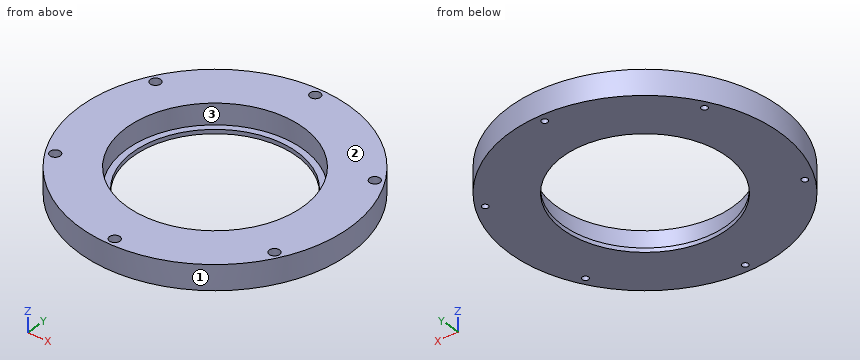
Autodesk Fusion 360 part; units mm, degrees
sketch "Sketch1" plane through (0, 0, 0) normal (0, 0, 1) x (1, 0, 0)
  circle A0 centre (0, 0) radius 65
  circle A1 centre (0, 0) radius 61.0225 construction
  circle A2 centre (0, 0) radius 39.5
  circle A3 centre (0, -61.0225) radius 1.5
  dimension "d1" = 130
  dimension "d2" = 122.045
  dimension "d3" = 79
  dimension "ScrewDia" = 3
extrude "Extrude1" add sketch "Sketch1" along normal blind 2 contours A0 | A3
sketch "Sketch2" plane through (0, 0, 2) normal (0, 0, 1) x (-1, 0, 0)
  circle A0 centre (0, 0) radius 39.5
  circle A1 centre (0, 0) radius 65
  circle A2 centre (0, 0) radius 42.5
  dimension "BearingDia" = 85
extrude "Extrude2" add sketch "Sketch2" along normal blind 10 contours A1
extrude "Extrude3" cut sketch "Sketch1" along normal blind 25 contours A3
sketch "Sketch3" plane through (0, 0, 12) normal (0, 0, 1) x (-1, 0, 0)
  circle A0 centre (0, 61.0225) radius 1.5
  circle A1 centre (0, 0) radius 42.5
  circle A2 centre (0, 0) radius 65
  circle A3 centre (0, -61.0225) radius 2.5
  dimension "ScrewHeadDia" = 5
extrude "Extrude4" cut sketch "Sketch3" against normal blind 5 contours A3
pattern_circular "C-Pattern1" count 6 over 360 about axis through (0, 0, 1.75) along (0, 0, 1) of "Extrude3", "Extrude4"
Input: part model. Units: mm. Frame: model coordinates. Face numbers are marked on the shaded views. Coordinates: 2 decimals unless noted, no trailing zeros. Loops run counter-clockwise (first coordinate to the right, second up) from the corner with the lowest first, then second, coordinate; pieces in that order, holes last.
Q1. Cut plane B-B (y = 0). Output: boundary loops of the cut face in (x, z), then the cut area to 3 significant figures.
Q2. Cut plane A-A (x = 0). Output: boundary loops of the cut face in (y, z), then the cut area to 3 significant figures.
Q3. Cut plane D-D (x = -41). Output: boundary loops of the cut face in (y, z), then the cut area to 3 significant figures.
Q4. Contact query for flat-ended pins moving along their axis: pin 1 (1.5 mm diameter, centred on x = 31, z = 3, fed in from -Y); pin 2 (1 mm diameter, centred on x = 12, z = 2.5, fed in from +Y); pin 3 (1.5 mm diameter, centred on x = -52, y = -30.5, fed in from +Z). Output: stop coordinate, or through.
Q5. Cut plane C-C (z = 5.5). Output: boundary loops of the cut face in (x, y), then the cut area to 3 significant figures.
Q6. Material intervals for line 1 (Y direction, x = 0, z = 1.05); line 2 (Y direction, x = 0, z = 5); line 3 (X direction, y = 0, z = 5), sorted ascending.
Q7. Draft query along X for the marked faces 1, 2 and 3. Return one class per face: +X half, -X half, draft (parallel to the pull), parting line (faces both ways), or undercut.
Working result:
1. outline: (-65, 0) - (-39.5, 0) - (-39.5, 2) - (-42.5, 2) - (-42.5, 12) - (-65, 12) - close; (39.5, 0) - (65, 0) - (65, 12) - (42.5, 12) - (42.5, 2) - (39.5, 2) - close
1. area: 552 mm2
2. outline: (-65, 0) - (-62.52, 0) - (-62.52, 7) - (-63.52, 7) - (-63.52, 12) - (-65, 12) - close; (-59.52, 0) - (-39.5, 0) - (-39.5, 2) - (-42.5, 2) - (-42.5, 12) - (-58.52, 12) - (-58.52, 7) - (-59.52, 7) - close; (39.5, 0) - (59.52, 0) - (59.52, 7) - (58.52, 7) - (58.52, 12) - (42.5, 12) - (42.5, 2) - (39.5, 2) - close; (62.52, 0) - (65, 0) - (65, 12) - (63.52, 12) - (63.52, 7) - (62.52, 7) - close
2. area: 460 mm2
3. outline: (-50.44, 0) - (50.44, 0) - (50.44, 12) - (11.19, 12) - (11.19, 2) - (-11.19, 2) - (-11.19, 12) - (-50.44, 12) - close
3. area: 987 mm2
4. pin 1: stops at y = -57.53
4. pin 2: stops at y = 63.97
4. pin 3: stops at z = 7
5. outline: circle Ø130 at (0, 0); hole circle Ø3 at (-52.85, -30.51); hole circle Ø3 at (-52.85, 30.51); hole circle Ø85 at (0, 0); hole circle Ø3 at (0, -61.02); hole circle Ø3 at (0, 61.02); hole circle Ø3 at (52.85, -30.51); hole circle Ø3 at (52.85, 30.51)
5. area: 7,560 mm2
6. line 1: y = -65 to -62.52, -59.52 to -39.5, 39.5 to 59.52, 62.52 to 65
6. line 2: y = -65 to -62.52, -59.52 to -42.5, 42.5 to 59.52, 62.52 to 65
6. line 3: x = -65 to -42.5, 42.5 to 65
7. face 1: parting line
7. face 2: draft
7. face 3: undercut
